Can you work these out from the model? Positions are in its coordinate system, mm. Face numbers are marked on the shaded views. A direction names the side the tool comes from. Coordinates: 2 decimals unless noted, no trailing zeros. Order: outer loops, then holes, each group sorted by start corner. A loop starts at its lowest first (then second) coordinate and runs counter-clockwise, first axis right, second up. Notation, with made-up numbers: M 89.5,58 L 95.5,58 A14 cw 95.5,71 Z; hole C -40,-0.75 d9. An arc over 180 degrees is marked long. Answer as CSV lines item,"result". Start each with the question number.
1. On a 3-axis mill with a long thin cutter (end or side, diameter ignored), from which of +Z, -Z, +X, -X, +Y, -Y can I reach the whole of each face in a straight line? I mean the marked faces 1 and 2. Say none if no direction works.
2. If we section it at C-C (x = 35.5): List the corners of the cut face in (y, z) for me, plus the area to 3 significant figures.
3. If we section it at A-A (z = 7): List the corners of the cut face in (x, y) for me, plus the area to 3 significant figures.
4. If we mould it in two halves opening along X, with no side actions, what happens to the marked faces 3, 4, 5 and 6? For each: released by +X, released by -X, zero draft, split by the parting line, or undercut.
5. I need wall thicknesses on line 1 along X through (y, z) = (34.5, 1.25); line 2 along Z through (x, y) = (8.5, 0.5); line 3 along X through (y, z) = (4.5, 11). Which ranges of each line are inside material? Lowest first, please. Write a range as from..to.
6. If we section it at D-D (x = 106.5): List the corners of the cut face in (y, z) for me, plus the area to 3 significant figures.
7. Will these pins go through, and if not, where does the flat tip stop? pin 1 (3 mm diameter, centred on x = 6.065, y = 5.395, fed in from +Z); pin 2 (8 mm diameter, centred on x = 55.5, y = 13.5, fed in from -Z); pin 3 (11.5 mm diameter, centred on x = 69.5, y = 26, fed in from +Z).
8. If we section it at B-B (y = 10): List the corners of the cut face in (x, z) for me, plus the area to 3 significant figures.
```python
from build123d import *

# Parameters (mm, degrees)
SKETCH_W        = 115
SKETCH_H        = 40
PAD_DEPTH       = 12
SKETCH001_W     = 112.6
SKETCH001_H     = 37.6
POCKET_DEPTH    = 11
SKETCH002_R     = 3.6
PAD001_DEPTH    = 2
SKETCH004_R     = 1.5
POCKET001_DEPTH = 115.001
FILLET_R        = 3
FILLET001_R     = 2
SKETCH011_R     = 1.5
POCKET006_DEPTH = 40.001
SKETCH012_R     = 1
POCKET007_DEPTH = 6


with BuildPart() as part:
    # Sketch → Pad (new body)
    with BuildSketch(Plane.XY):
        with Locations((57.5, 20)):
            Rectangle(SKETCH_W, SKETCH_H)
    extrude(amount=PAD_DEPTH)

    # Sketch001 (on Face6 of Pad) → Pocket (cut)
    with BuildSketch(Plane.XY.offset(12)):
        with Locations((57.5, 20)):
            Rectangle(SKETCH001_W, SKETCH001_H)
    extrude(amount=-POCKET_DEPTH, mode=Mode.SUBTRACT)

    # Sketch002 (on Face11 of Pocket) → Pad001 (join)
    with BuildSketch(Plane.XY.offset(1)):
        with Locations((6.065, 34.605)):
            Circle(SKETCH002_R)
        with Locations((6.065, 5.395)):
            Circle(SKETCH002_R)
        with Locations((108.935, 34.605)):
            Circle(SKETCH002_R)
        with Locations((108.935, 5.395)):
            Circle(SKETCH002_R)
    extrude(amount=PAD001_DEPTH)

    # Sketch004 (on Face2 of Pad001) → Pocket001 (cut, through all)
    with BuildSketch(Plane(origin=(0, 0, 0), x_dir=(0, -1, 0), z_dir=(-1, 0, 0))):
        with Locations((-32, 7)):
            Circle(SKETCH004_R)
    extrude(amount=-POCKET001_DEPTH, mode=Mode.SUBTRACT)

    # Fillet
    fillet_edges = [part.edges().sort_by_distance(p)[0] for p in [
        (1.2, 38.8, 6.5),
        (1.2, 1.2, 6.5),
        (113.8, 1.2, 6.5),
        (113.8, 38.8, 6.5),
    ]]
    fillet(fillet_edges, radius=FILLET_R)

    # Fillet001
    fillet001_edges = [part.edges().sort_by_distance(p)[0] for p in [
        (115, 0, 6),
        (115, 40, 6),
        (0, 40, 6),
        (0, 0, 6),
    ]]
    fillet(fillet001_edges, radius=FILLET001_R)

    # Sketch011 (on Face2 of Fillet001) → Pocket006 (cut, through all)
    with BuildSketch(Plane.XZ):
        with Locations((8.5, 9.6)):
            Circle(SKETCH011_R)
        with Locations((106.5, 9.6)):
            Circle(SKETCH011_R)
    extrude(amount=-POCKET006_DEPTH, mode=Mode.SUBTRACT)

    # Sketch012 (on Face32 of Pocket006) → Pocket007 (cut)
    with BuildSketch(Plane.XY.offset(3)):
        with Locations((6.065, 34.605)):
            Circle(SKETCH012_R)
        with Locations((108.935, 34.605)):
            Circle(SKETCH012_R)
        with Locations((108.935, 5.395)):
            Circle(SKETCH012_R)
        with Locations((6.065, 5.395)):
            Circle(SKETCH012_R)
    extrude(amount=-POCKET007_DEPTH, mode=Mode.SUBTRACT)


solid = part.part
```
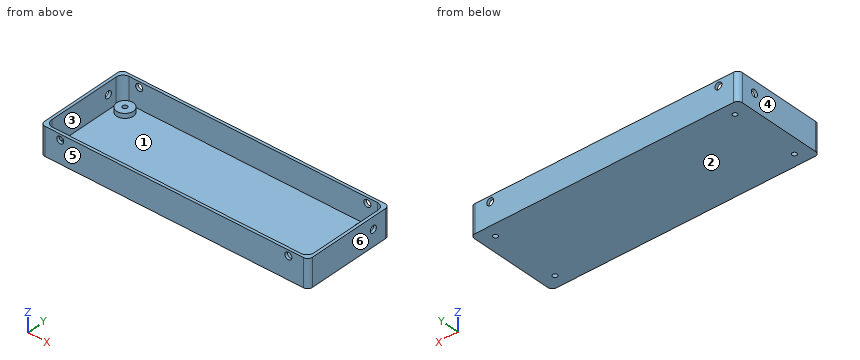
Solved:
1,face 1,"+Z"
1,face 2,"-Z, +X, -X, +Y, -Y"
2,outline,"M 0,0 L 40,0 L 40,12 L 38.8,12 L 38.8,1 L 1.2,1 L 1.2,12 L 0,12 Z"
2,area,"66.4 mm²"
3,outline,"M 0,2 A2 ccw 2,0 L 113,0 A2 ccw 115,2 L 115,30.5 L 113.8,30.5 L 113.8,4.2 A3 cw 110.8,1.2 L 4.2,1.2 A3 cw 1.2,4.2 L 1.2,30.5 L 0,30.5 Z; M 0,33.5 L 1.2,33.5 L 1.2,35.8 A3 cw 4.2,38.8 L 110.8,38.8 A3 cw 113.8,35.8 L 113.8,33.5 L 115,33.5 L 115,38 A2 ccw 113,40 L 2,40 A2 ccw 0,38 Z"
3,area,"363 mm²"
4,face 3,"undercut"
4,face 4,"released by -X"
4,face 5,"zero draft"
4,face 6,"released by +X"
5,line 1,"0..1.2, 2.47..5.07, 7.06..9.66, 105.34..107.94, 109.93..112.53, 113.8..115"
5,line 2,"0..8.1, 11.1..12"
5,line 3,"0..1.2, 113.8..115"
6,outline,"M 0,0 L 40,0 L 40,8.1 L 38.8,8.1 L 38.8,1 L 37.26,1 L 37.26,3 L 31.95,3 L 31.95,1 L 8.05,1 L 8.05,3 L 2.74,3 L 2.74,1 L 1.2,1 L 1.2,8.1 L 0,8.1 Z; M 0,11.1 L 1.2,11.1 L 1.2,12 L 0,12 Z; M 38.8,11.1 L 40,11.1 L 40,12 L 38.8,12 Z"
6,area,"80.4 mm²"
7,pin 1,"z = 3"
7,pin 2,"z = 0"
7,pin 3,"z = 1"
8,outline,"M 0,0 L 115,0 L 115,12 L 113.8,12 L 113.8,1 L 1.2,1 L 1.2,12 L 0,12 Z"
8,area,"141 mm²"
